Part model, mm, in its own coordinate system. A direction names the side the tool comes from. Give positions to 0.01 mm unless a question says otherwise; leave off trailing zeros. Loops run counter-clockwise (first coordinate to the right, second up) from the corner with the lowest first, then second, coordinate; pieces in that order, holes last. Notation, with made-up numbers: M -20,89.5 L 21,89.5 A35 cw 21,128.5 Z; hole C 59,-34.75 d6. An arc over 180 degrees is marked long. Answer in a Markdown table with one row per item.
from build123d import *

# Parameters (mm, degrees)
BODYSKE_R   = 2
BODYSKE_R_2 = 0.45
BODYSKE_R_3 = 0.6
BODY_DEPTH  = 5
BOXSKE_R    = 1.4
BOX_DEPTH   = 3.9
HOLESKE_R   = 2.35
HOLE_DEPTH  = 21.081085628
PADSKE_R    = 3
PAD_DEPTH   = 0.5


with BuildPart() as part:
    # BodySke → Body (new, symmetric)
    with BuildSketch(Plane.XY):
        with BuildLine():
            Line((-3, 6), (13.5, 6))
            ThreePointArc((13.5, 6), (14.207106781, 5.707106781), (14.5, 5))
            Line((14.5, 5), (14.5, -5))
            ThreePointArc((14.5, -5), (14.207106781, -5.707106781), (13.5, -6))
            Line((13.5, -6), (-3, -6))
            ThreePointArc((-3, -6), (-3.707106781, -5.707106781), (-4, -5))
            Line((-4, -5), (-4, 5))
            ThreePointArc((-4, 5), (-3.707106781, 5.707106781), (-3, 6))
        make_face()
        Circle(BODYSKE_R, mode=Mode.SUBTRACT)
        with Locations((5, 0)):
            Circle(BODYSKE_R_2, mode=Mode.SUBTRACT)
        with Locations((-2.504495957, 4.5)):
            Circle(BODYSKE_R_3, mode=Mode.SUBTRACT)
        with Locations((-2.504495957, -4.5)):
            Circle(BODYSKE_R_3, mode=Mode.SUBTRACT)
        with Locations((6.175559685, 3.136966596)):
            Circle(BODYSKE_R_2, mode=Mode.SUBTRACT)
        with Locations((9.5, 3.55)):
            Circle(BODYSKE_R_2, mode=Mode.SUBTRACT)
        with Locations((9.595504043, -4.5)):
            Circle(BODYSKE_R_3, mode=Mode.SUBTRACT)
    extrude(amount=BODY_DEPTH, both=True)

    # BoxSke → Box (cut, symmetric)
    with BuildSketch(Plane.XY):
        with BuildLine():
            Line((12, 6), (12, -6))
            Line((12, -6), (-1.004495957, -6))
            Line((-1.004495957, -6), (-1.004495957, -4.5))
            ThreePointArc((-1.004495957, -4.5), (-1.443835785, -3.439339828), (-2.504495957, -3))
            Line((-2.504495957, -3), (-4, -3))
            Line((-4, -3), (-4, 3))
            Line((-4, 3), (-2.504495957, 3))
            ThreePointArc((-2.504495957, 3), (-1.443835785, 3.439339828), (-1.004495957, 4.5))
            Line((-1.004495957, 4.5), (-1.004495957, 6))
            Line((-1.004495957, 6), (12, 6))
        make_face()
        with Locations((9.595504043, -4.5)):
            Circle(BOXSKE_R, mode=Mode.SUBTRACT)
    extrude(amount=BOX_DEPTH, both=True, mode=Mode.SUBTRACT)

    # HoleSke → Hole (cut, through all)
    with BuildSketch(Plane(origin=(14.5, 0, 0), x_dir=(0, 0, -1), z_dir=(1, 0, 0))):
        Circle(HOLESKE_R)
    extrude(amount=-HOLE_DEPTH, mode=Mode.SUBTRACT)

    # PadSke → Pad (cut)
    with BuildSketch(Plane(origin=(14.5, 0, 0), x_dir=(0, 0, -1), z_dir=(1, 0, 0))):
        Circle(PADSKE_R)
    extrude(amount=-PAD_DEPTH, mode=Mode.SUBTRACT)


solid = part.part
(1) Saw through at B-B (x = 11.25). Write the cut outline in (y, z), plus the area to 3 significant figures.
Recorded:
| item | result |
|---|---|
| outline | M -6,-5 L 6,-5 L 6,-3.9 L -6,-3.9 Z; M -6,3.9 L 6,3.9 L 6,5 L -6,5 Z |
| area | 26.4 mm^2 |
(2) Drill centre lines: line 1 along X through (y, z) = (0, -4.15); line 2 along Z through (x, y) = (8, 2); line 3 along X through (y, z) = (4.75, 2.5). Where is each one in solid material? Low to high.
Recorded:
| item | result |
|---|---|
| line 1 | x = -4 to -2, 2 to 4.55, 5.45 to 14.5 |
| line 2 | z = -5 to -3.9, 3.9 to 5 |
| line 3 | x = -4 to -3.05, -1.96 to -1, 12 to 14.5 |
(3) Saw through at D-D (x = 0). Write the cut outline in (y, z).
Recorded:
| item | result |
|---|---|
| outline | M -6,-5 L -2,-5 L -2,-3.9 L -6,-3.9 Z; M -6,3.9 L -2,3.9 L -2,5 L -6,5 Z; M 2,-5 L 6,-5 L 6,-3.9 L 2,-3.9 Z; M 2,3.9 L 6,3.9 L 6,5 L 2,5 Z |
(4) Pin check, flat tip, straight feed: pin 1 Ø1.2 at (x, z) = (-3.5, -0.5) entering from -Y. Stop position of the tip, or through.
Recorded:
| item | result |
|---|---|
| pin 1 | stops at y = -6 |
(5) Saw through at A-A (z = 0). Give the number of separate pieces and of enclosed holes in the cut face, plus the area to 3 significant figures.
Recorded:
| item | result |
|---|---|
| separate pieces | 5 |
| enclosed holes | 3 |
| area | 36.5 mm^2 |
(6) Which spindle directions (+Z, -Z, +X, -X, +Y, -Y) get a long thin tool onto all of the face, cutting with end or side? Do faces 1 (the face through (5.4, -6, -4.4)), 2 (the face through (8.485, -5.352, -0.055)), 3 (the face through (-3, 3, 0)). Say none if no direction does.
Recorded:
| item | result |
|---|---|
| face 1 | +Z, -Z, +X, -X, -Y |
| face 2 | none |
| face 3 | -X |
(7) Pull direction X, two halves, no side cores. Call faces 4 (the face through (-4, -3.4, 0.1)), 5 (the face through (-3, -3, 0)), 6 (the face through (14.215, -5.699, 0.07)), 7 (the face through (8.996, -4.474, -0.07)): +X half, -X half, draft (parallel to the pull), parting line (faces both ways), or undercut.
Recorded:
| item | result |
|---|---|
| face 4 | -X half |
| face 5 | draft |
| face 6 | +X half |
| face 7 | undercut |
